The model under review builds one solid part; all positions refer to its coordinate system, in mm. Round coordinates to 2 decimals unless told otherwise and drop trailing zeros. Write each loop counter-clockwise with the first axis right and the second up, starting at its lowest first coordinate (ties: lowest second). Pieces come first, ordered by that corner, then holes. Notation, with made-up numbers: (71.5, -13.5) - (88.5, -13.5) arc R33 ccw to (88.5, 19.5) - close; hole circle Ø10 at (23, 55.25). An arc over 180 degrees is marked (long way). Return JSON: item names as keys, results as strings.
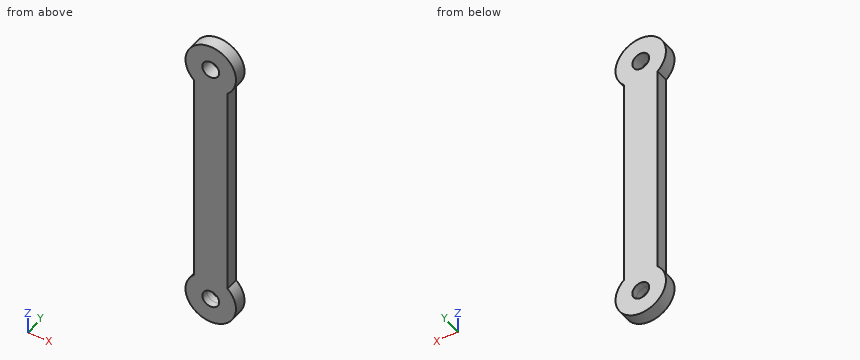
from build123d import *

# Parameters (mm, degrees)
F1_DEPTH = 4


with BuildPart() as f1:
    # F0 (on Front) → F1 (new body, symmetric)
    with BuildSketch(Plane.XZ):
        with BuildLine():
            ThreePointArc((10, -11.1803398875), (13.6930639376, -6.123724357), (15, 0))
            ThreePointArc((15, 0), (6.123724357, 13.6930639376), (-10, 11.1803398875))
            Line((-10, 11.1803398875), (-10, -11.1803398875))
            ThreePointArc((-10, -11.1803398875), (-5.3523313466, -14.0125853844), (0, -15))
            ThreePointArc((0, -15), (5.3523313466, -14.0125853844), (10, -11.1803398875))
        make_face()
        with BuildLine():
            ThreePointArc((5, 0), (3.5355339059, -3.5355339059), (0, -5))
            ThreePointArc((0, -5), (-3.5355339059, 3.5355339059), (5, 0))
        make_face(mode=Mode.SUBTRACT)
        with BuildLine():
            Line((-10, -11.1803398875), (-10, 11.1803398875))
            ThreePointArc((-10, 11.1803398875), (-15, 0), (-10, -11.1803398875))
        make_face()
        with BuildLine():
            Line((10, -138.8196601125), (10, -11.1803398875))
            ThreePointArc((10, -11.1803398875), (5.3523313466, -14.0125853844), (0, -15))
            Line((0, -15), (0, -135))
            ThreePointArc((0, -135), (5.3523313466, -135.9874146156), (10, -138.8196601125))
        make_face()
        with BuildLine():
            ThreePointArc((0, -15), (-5.3523313466, -14.0125853844), (-10, -11.1803398875))
            Line((-10, -11.1803398875), (-10, -138.8196601125))
            ThreePointArc((-10, -138.8196601125), (-5.3523313466, -135.9874146156), (0, -135))
            Line((0, -135), (0, -15))
        make_face()
        with BuildLine():
            ThreePointArc((15, -150), (13.6930639376, -143.876275643), (10, -138.8196601125))
            ThreePointArc((10, -138.8196601125), (5.3523313466, -135.9874146156), (0, -135))
            ThreePointArc((0, -135), (-5.3523313466, -135.9874146156), (-10, -138.8196601125))
            ThreePointArc((-10, -138.8196601125), (-6.123724357, -163.6930639376), (15, -150))
        make_face()
        with BuildLine():
            ThreePointArc((5, -150), (-3.5355339059, -153.5355339059), (0, -145))
            ThreePointArc((0, -145), (3.5355339059, -146.4644660941), (5, -150))
        make_face(mode=Mode.SUBTRACT)
    extrude(amount=F1_DEPTH, both=True)


solid = f1.part
(1) Add section B-B (y = 2.5). Write out the cut boundary in (x, z).
Filled in:
{"outline": "(-10, -138.82) arc R15 ccw (long way) to (10, -138.82) - (10, -11.18) arc R15 ccw (long way) to (-10, -11.18) - close; hole circle Ø10 at (0, -150); hole circle Ø10 at (0, 0)"}
(2) Add section D-D (z = -111). Write out the cut boundary in (x, y).
Filled in:
{"outline": "(-10, -4) - (10, -4) - (10, 4) - (-10, 4) - close"}
(3) Add section A-A (z = 0). Write out the cut boundary in (x, y).
Filled in:
{"outline": "(-15, -4) - (-5, -4) - (-5, 4) - (-15, 4) - close; (5, -4) - (15, -4) - (15, 4) - (5, 4) - close"}
(4) Wall thickness on line 1 (X direction, y = 1.4, z = -150); line 2 (Z direction, x = 3, y = 3); line 3 (Z direction, x = 2.5, y = -1.25): over which ranges is each line inside the solid? List them lowest first.
Filled in:
{"line 1": "x = -15 to -5, 5 to 15", "line 2": "z = -164.7 to -154, -146 to -4, 4 to 14.7", "line 3": "z = -164.79 to -154.33, -145.67 to -4.33, 4.33 to 14.79"}
(5) Add section C-C (x = 3). Write out the cut boundary in (y, z), plus the area to 3 significant figures.
Filled in:
{"outline": "(-4, -164.7) - (4, -164.7) - (4, -154) - (-4, -154) - close; (-4, -146) - (4, -146) - (4, -4) - (-4, -4) - close; (-4, 4) - (4, 4) - (4, 14.7) - (-4, 14.7) - close", "area": "1,310 mm2"}
(6) Clearance check with flat-ended pins moving along their axes: pin 1 Ø2.5 at (y, z) = (1.5, -49.5) entering from +X; pin 2 Ø2.5 at (y, z) = (1, -77) entering from -X. State where each tip first meets the part, or that it passes through.
Filled in:
{"pin 1": "stops at x = 10", "pin 2": "stops at x = -10"}
